Drawing for the job (mm, zero at the part's lowest x, y, z). Give positions to 0.01 mm unless a question says otherwise; leave off trailing zeros. Order: outer loops, then holes, each group sorted by start corner. A loop starts at its lowest first (then second) coordinate and runs counter-clockwise, first axis right, second up. Notation, with made-up numbers: (-1, 29) - (41, 29) arc R26 ccw to (41, 54) - close; hole circle Ø9 at (41.5, 28). An arc over 180 degrees is marked (long way). One line per item, written item: value.
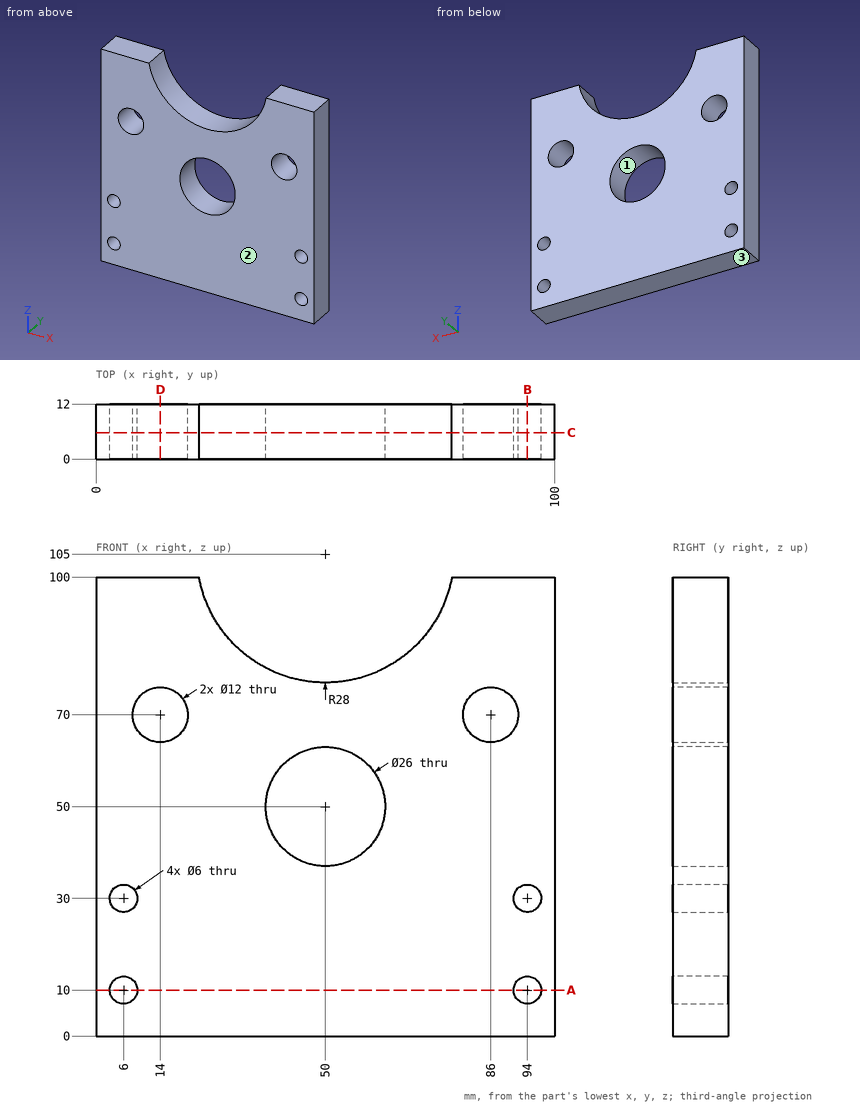
1) Cut at D-D, the plane x = 14. Give the cut face in (y, z), then the cut area to 3 significant figures.
Outcome:
outline: (0, 0) - (12, 0) - (12, 64) - (0, 64) - close; (0, 76) - (12, 76) - (12, 100) - (0, 100) - close
area: 1,060 mm^2
2) Cut at A-A, the plane z = 10. Give the cut face in (x, y).
Outcome:
outline: (0, 0) - (3, 0) - (3, 12) - (0, 12) - close; (9, 0) - (91, 0) - (91, 12) - (9, 12) - close; (97, 0) - (100, 0) - (100, 12) - (97, 12) - close
3) Cut at B-B, the plane x = 94. Give the cut face in (y, z).
Outcome:
outline: (0, 0) - (12, 0) - (12, 7) - (0, 7) - close; (0, 13) - (12, 13) - (12, 27) - (0, 27) - close; (0, 33) - (12, 33) - (12, 100) - (0, 100) - close
4) Mould opens along Z. For the marked faces 1, 2 and 3 say: released by +Z, released by -Z, zero draft, split by the parting line, or undercut.
Outcome:
face 1: undercut
face 2: zero draft
face 3: released by -Z
5) Drill centre lines: line 1 along X through (y, z) = (0.75, 67); line 2 along X through (y, z) = (1, 50.5); line 3 along X through (y, z) = (4.5, 9). Where is each one in solid material? Low to high. Write a range as from..to.
Outcome:
line 1: x = 0..8.8, 19.2..80.8, 91.2..100
line 2: x = 0..37.01, 62.99..100
line 3: x = 0..3.17, 8.83..91.17, 96.83..100
6) Cut at C-C, the plane y = 5.75. Give the cut face in (x, z), then the cut area to 3 significant figures.
Outcome:
outline: (0, 0) - (100, 0) - (100, 100) - (77.55, 100) arc R28 cw to (22.45, 100) - (0, 100) - close; hole circle Ø6 at (6, 10); hole circle Ø6 at (6, 30); hole circle Ø12 at (14, 70); hole circle Ø26 at (50, 50); hole circle Ø12 at (86, 70); hole circle Ø6 at (94, 10); hole circle Ø6 at (94, 30)
area: 8,180 mm^2
